from build123d import *

# Parameters (mm, degrees)
F0_R             = 53.5
F0_R_2           = 36.5
F1_DEPTH         = 15
F5_D             = 6
F5_CBORE_D       = 9
F5_CBORE_DEPTH   = 5
F7_W             = 14
F7_H             = 11
F8_DEPTH         = 15
F10_W            = 14
F10_H            = 11
F11_DEPTH        = 15
F13_R            = 2.05
F14_DEPTH        = 2.2
F16_R            = 2.05
F17_DEPTH        = 2.2
F18_R            = 3
F19_DEPTH        = 7.5
F20_DEPTH        = 7.5
F21_R            = 3
F22_R            = 3
F25_W            = 4
F25_H            = 7.5
F26_DEPTH        = 1.5
F26_COPIES_COUNT = 4
F27_R            = 0.5
F29_D            = 1.5


# Not quite as in the source:
# - a pattern or mirror of a feature is missing from the dataset's text; its kind, count and spacing are read off the source's solid


with BuildPart() as f1:
    # F0 (on Top) → F1 (new body)
    with BuildSketch(Plane.XY):
        Circle(F0_R)
        Circle(F0_R_2, mode=Mode.SUBTRACT)
    extrude(amount=F1_DEPTH)

    # F5 (through all)
    with Locations(Plane.XY.offset(15)):
        with Locations((-31.8198051534, 31.8198051534), (31.8198051534, -31.8198051534)):
            CounterBoreHole(F5_D / 2, F5_CBORE_D / 2, F5_CBORE_DEPTH)

    # F7 (on plane+point) → F8 (cut)
    with BuildSketch(Plane.XZ.offset(-33.5)):
        with Locations((0, 9.5)):
            Rectangle(F7_W, F7_H)
    extrude(amount=-F8_DEPTH, mode=Mode.SUBTRACT)

    # F10 (on plane+point) → F11 (cut)
    with BuildSketch(Plane.XZ.offset(33.5)):
        with Locations((0, 9.5)):
            Rectangle(F10_W, F10_H)
    extrude(amount=F11_DEPTH, mode=Mode.SUBTRACT)

    # F13 (on plane+point) → F14 (cut)
    with BuildSketch(Plane.XZ.offset(53.5)):
        with Locations((0, 8)):
            Circle(F13_R)
    extrude(amount=-F14_DEPTH, mode=Mode.SUBTRACT)

    # F16 (on plane+point) → F17 (cut)
    with BuildSketch(Plane.XZ.offset(-53.5)):
        with Locations((0, 8)):
            Circle(F16_R)
    extrude(amount=F17_DEPTH, mode=Mode.SUBTRACT)

    # F18 (on face) → F19 (cut)
    with BuildSketch(Plane(origin=(0, 0, 0), x_dir=(1, 0, 0), z_dir=(0, 0, -1))):
        Polygon((-33.2340187158, -24.0416305603), (-39.5979797464, -30.405591591), (-30.405591591, -39.5979797464), (-24.0416305603, -33.2340187158), align=None)
        with Locations((-31.8198051534, -31.8198051534)):
            Circle(F18_R, mode=Mode.SUBTRACT)
    extrude(amount=-F19_DEPTH, mode=Mode.SUBTRACT)

    # F18 (on face) → F20 (cut)
    with BuildSketch(Plane(origin=(0, 0, 0), x_dir=(1, 0, 0), z_dir=(0, 0, -1))):
        Polygon((-33.2340187158, -24.0416305603), (-39.5979797464, -30.405591591), (-30.405591591, -39.5979797464), (-24.0416305603, -33.2340187158), align=None)
        Polygon((30.405591591, 39.5979797464), (24.0416305603, 33.2340187158), (33.2340187158, 24.0416305603), (39.5979797464, 30.405591591), align=None)
    extrude(amount=-F20_DEPTH, mode=Mode.SUBTRACT)

    # F21
    f21_edges = [f1.edges().sort_by_distance(p)[0] for p in [
        (-36.5, 0, 15),
    ]]
    fillet(f21_edges, radius=F21_R)

    # F22
    f22_edges = [f1.edges().sort_by_distance(p)[0] for p in [
        (-53.5, 0, 15),
        (28.175787, 23.202909, 15),
        (28.175787, -23.202909, 15),
    ]]
    fillet(f22_edges, radius=F22_R)

    # F25 (on face) → F26 (join, symmetric)
    with BuildSketch(Plane(origin=(37.8302127935, 37.8302127935, 0), x_dir=(-0.7071067812, 0.7071067812, 0), z_dir=(0.7071067812, 0.7071067812, 0))):
        with Locations((0, 8.25)):
            Rectangle(F25_W, F25_H)
    f26 = extrude(amount=F26_DEPTH, both=True)

    # F26_copies: F26 ×4 about axis
    f26_copies_axis = Axis((0, 0, 0), (0, 0, 1))
    for i in range(1, F26_COPIES_COUNT):
        add(f26.rotate(f26_copies_axis, i * 360 / F26_COPIES_COUNT))

    # F27
    f27_edges = [f1.edges().sort_by_distance(p)[0] for p in [
        (39.217983, 36.389556, 8.25),
        (36.389556, 39.217983, 8.25),
        (37.830213, 37.830213, 4.5),
        (39.217983, -36.389556, 8.25),
        (37.830213, -37.830213, 4.5),
        (36.389556, -39.217983, 8.25),
        (-36.389556, -39.217983, 8.25),
        (-37.830213, -37.830213, 4.5),
        (-39.217983, -36.389556, 8.25),
        (-39.217983, 36.389556, 8.25),
        (-37.830213, 37.830213, 4.5),
        (-36.389556, 39.217983, 8.25),
    ]]
    fillet(f27_edges, radius=F27_R)

    # F29 (through all)
    with Locations(Plane(origin=(0, 51.3, 0), x_dir=(-1, 0, 0), z_dir=(0, 1, 0))):
        with Locations((0, 8)):
            Hole(F29_D / 2)


solid = f1.part
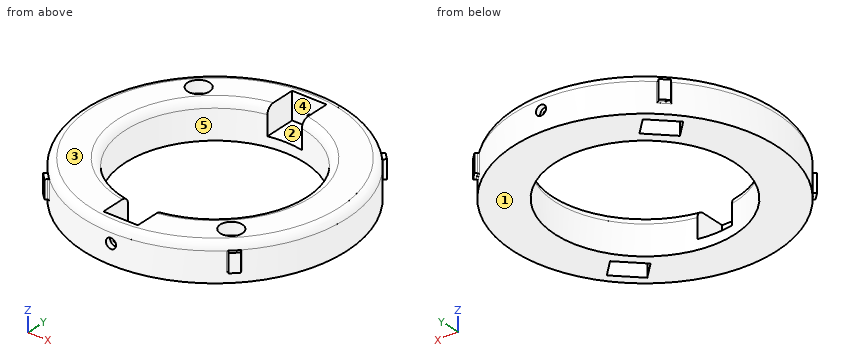
Could you check a few things on this model? Use its own coordinates, in mm. Face numbers are marked on the shaded views. A direction names the side the tool comes from. Give positions to 0.01 mm unless a question says otherwise; leave off trailing zeros. Order: outer loops, then holes, each group sorted by start corner. A loop starts at its lowest first (then second) coordinate and runs counter-clockwise, first axis right, second up.
1. Will these pins go through, and if not, where does the flat tip stop? P1, Ø8, axis at x = 31.82, y = -31.82, coming from the +Z side; P2, Ø1.8, axis at x = -39, y = -39, coming from the -Z side; P3, Ø1, axis at x = -40, z = 9.5, coming from the +Y side.
2. I need wall thicknesses on L1, parallel to Z at x = 0, y = 49.4; L2, parallel to X at y = -28.5, z = 11.75; L3, parallel to Y at x = 32, z = 1.5. Which ranges of each line are inside material? Lowest first, please.
3. For the marked faces 1 and 2, which set-ups out of +Z, -Z, +X, -X, +Y, -Y let a thin tool reach every point of the face, with its end or its side?
4. Suppose I cut it at A-A (z = 2.25). List the corners of the cut face in (x, y) for me, plus the area to 3 significant figures.
5. We'd pull the mould along Y, two halves only. Please class the marked faces 3, 4 and 5: pulls with the +Y half, pulls with the -Y half, needs draft (parallel to the pull), parting line crosses it, or undercut.
Solved:
1. P1: stops at z = 10
1. P2: stops at z = 4.5
1. P3: stops at y = 38.28
2. L1: z = 0 to 7.25, 8.75 to 15
2. L2: x = -45.28 to -22.8, 22.8 to 28.78, 34.86 to 45.28
2. L3: y = -42.87 to -38, -25.28 to -17.56, 17.56 to 42.87
3. face 1: -Z, +X, -X, +Y, -Y
3. face 2: +Z
4. outline: circle Ø107 at (0, 0); hole (-39.6, 30.41) - (-33.23, 24.04) - (-24.04, 33.23) - (-30.41, 39.6) - close; hole circle Ø73 at (0, 0); hole (24.04, -33.23) - (30.41, -39.6) - (39.6, -30.41) - (33.23, -24.04) - close
4. area: 4,570 mm2
5. face 3: needs draft
5. face 4: undercut
5. face 5: undercut
